The listing builds one solid part. Answer for the finished solid, in the listing's coordinates (mm). A direction names the side the tool comes from. Coordinates: 2 decimals unless noted, no trailing zeros. Order: outer loops, then holes, each group sorted by start corner. A loop starts at its lowest first (then second) coordinate and runs counter-clockwise, first axis right, second up. Notation, with made-up numbers: (77.5, 75.25) - (93.5, 75.25) arc R15 ccw to (93.5, 98.25) - close; hole circle Ø2 at (76.25, -30). An arc over 180 degrees is marked (long way). Use a Markdown table: item, result. Add a question column.
Item 1: Find the intervals of material crossed by line 1 along X through (y, z) = (-6.75, -6.5); line 2 along X through (y, z) = (-0.5, -10); line 3 along Z through (x, y) = (-9, 16.75), in increasing order.
Item 2: Flat-ended cylindrical pins translate along their axes: P1, Ø2, axis at x = -8.5, y = -4.5, coming from the -Z side; P2, Ø5, axis at x = -2, z = -6.5, coming from the +Y side; P3, Ø4, axis at x = 9.5, z = -1, coming from the -Y side; P4, Ø2, axis at y = 11.5, z = 0.5, coming from the -X side. Find the tip coordinate at first contact, or state that the pin passes through.
Item 3: The part is cut by section C-C, the plane x = 11.5. Give the vertices of the cut face in (y, z).
Item 4: The part is cut by section D-D, the plane z = -3. Give the vertices of the cut face in (x, y).
Item 5: The part is cut by section A-A, the plane y = 11. Give the vertices of the cut face in (x, z).
Item 6: For faces 4 (the flat face through (14.99, -0.83, -2.73)), 5 (the flat face through (19.014, -7, -3)), 6 (the flat face through (11.014, -7, -3)), 7 (the flat face through (12, -6.45, -3)), determine the directions among +Z, -Z, +X, -X, +Y, -Y from which every point of the face is accessible in a straight line to the end or side of a thin tool.
Item 7: The mould has two halves that part along X. Classify faces 1 (the flat face through (-10, -7, -8)), 2 (the flat face through (18.014, 9, 0)), 3 (the flat face through (8.989, 18.924, 0.479)): released by +X, released by -X, zero draft, split by the parting line, or undercut.
Item 8: The part is cut by section B-B, the plane z = -0.25. Give the vertices of the cut face in (x, y) (3 decimals).
from build123d import *

# Parameters (mm, degrees)
EXTRUDE_1_DEPTH      = 2
EXTRUDE_1_DEPTH_BACK = 1
BOSS_EXTRUDE1_DEPTH  = 10
LPATTERN1_COUNT      = 2
LPATTERN1_PITCH      = 25
SKETCH2_W            = 3
SKETCH2_H            = 4
BOSS_EXTRUDE2_DEPTH  = 14
BOSS_EXTRUDE3_DEPTH  = 4
LPATTERN2_COUNT      = 2
LPATTERN2_PITCH      = 25
CUT_EXTRUDE1_DEPTH   = 10


with BuildPart() as part:
    # Эскиз2 → Бобышка-Вытянуть1 (new, two sides: drawn at the far end of the back side and taken through both)
    with BuildSketch(Plane.XY.offset(-EXTRUDE_1_DEPTH_BACK)):
        Polygon((18.01429863, 0), (18.01429863, 26.7), (-11.98570137, 26.7), (-11.98570137, -2.25), (18.01429863, -2.25), align=None)
    extrude(amount=EXTRUDE_1_DEPTH + EXTRUDE_1_DEPTH_BACK)

    # Sketch1 → Boss-Extrude1 (add)
    with BuildSketch(Plane.XY.offset(2)):
        with BuildLine():
            Line((-5.98570137, -6.45), (-7.98570137, -6.45))
            Line((-7.98570137, -6.45), (-7.98570137, -2.25))
            Line((-7.98570137, -2.25), (-11.98570137, -2.25))
            Line((-11.98570137, -2.25), (-11.98570137, -6.45))
            Line((-11.98570137, -6.45), (-13.98570137, -6.45))
            Line((-13.98570137, -6.45), (-13.98570137, -7.45))
            ThreePointArc((-13.98570137, -7.45), (-13.399914932, -8.864213562), (-11.98570137, -9.45))
            Line((-11.98570137, -9.45), (-7.98570137, -9.45))
            ThreePointArc((-7.98570137, -9.45), (-6.571487808, -8.864213562), (-5.98570137, -7.45))
            Line((-5.98570137, -7.45), (-5.98570137, -6.45))
        make_face()
    boss_extrude1 = extrude(amount=-BOSS_EXTRUDE1_DEPTH)

    # LPattern1: Boss-Extrude1 ×2
    with Locations(*[(i * LPATTERN1_PITCH, 0, 0) for i in range(1, LPATTERN1_COUNT)]):
        add(boss_extrude1)

    # Sketch2 → Boss-Extrude2 (add)
    with BuildSketch(Plane(origin=(0, 0, 2), x_dir=(-1, 0, 0), z_dir=(0, 0, -1))):
        with Locations((-9.283605158, -0.25)):
            Rectangle(SKETCH2_W, SKETCH2_H)
    extrude(amount=BOSS_EXTRUDE2_DEPTH)

    # Sketch3 → Boss-Extrude3 (add)
    with BuildSketch(Plane.ZY.offset(-13.01429863)):
        Polygon((-4.5, -2.25), (-1, -2.25), (-1, 0.558861968), align=None)
    boss_extrude3 = extrude(amount=-BOSS_EXTRUDE3_DEPTH)

    # LPattern2: Boss-Extrude3 ×2
    with Locations(*[(-i * LPATTERN2_PITCH, 0, 0) for i in range(1, LPATTERN2_COUNT)]):
        add(boss_extrude3)

    # Sketch4 → Cut-Extrude1 (cut)
    with BuildSketch(Plane(origin=(0, 0, -1), x_dir=(-1, 0, 0), z_dir=(0, 0, -1))):
        with BuildLine():
            Line((-10.321327868, 19.682942102), (-7.619737196, 18.144453997))
            ThreePointArc((-7.619737196, 18.144453997), (-9.751909083, 15.519632814), (-10.51429863, 12.225))
            ThreePointArc((-10.51429863, 12.225), (-3.01429863, 4.725), (4.48570137, 12.225))
            ThreePointArc((4.48570137, 12.225), (3.723311823, 15.519632814), (1.591139935, 18.144453997))
            Line((1.591139935, 18.144453997), (4.292730608, 19.682942102))
            Line((4.292730608, 19.682942102), (13.385264368, 19.682942102))
            Line((13.385264368, 19.682942102), (19.56091022, 30.423181844))
            Line((19.56091022, 30.423181844), (-22.587954431, 29.74009492))
            Line((-22.587954431, 29.74009492), (-18.01429863, 19.682942102))
            Line((-18.01429863, 19.682942102), (-10.321327868, 19.682942102))
        make_face()
    extrude(amount=-CUT_EXTRUDE1_DEPTH, mode=Mode.SUBTRACT)


solid = part.part
Solution:
| question | item | result |
|---|---|---|
| 1 | line 1 | x = -13.99 to -5.99, 11.01 to 19.01 |
| 1 | line 2 | x = 7.78 to 10.78 |
| 1 | line 3 | z = -1 to 2 |
| 2 | P1 | stops at z = -8 |
| 2 | P2 | passes through |
| 2 | P3 | stops at y = -8.76 |
| 2 | P4 | stops at x = -11.99 |
| 3 | outline | (-8.76, -8) - (-6.45, -8) - (-6.45, 2) - (-8.76, 2) - close; (-2.25, -1) - (19.68, -1) - (19.68, 2) - (-2.25, 2) - close |
| 4 | outline | (-13.99, -7.45) arc R2 ccw to (-11.99, -9.45) - (-7.99, -9.45) arc R2 ccw to (-5.99, -7.45) - (-5.99, -6.45) - (-7.99, -6.45) - (-7.99, -1.05) - (-11.99, -1.05) - (-11.99, -6.45) - (-13.99, -6.45) - close; (7.78, -2.25) - (10.78, -2.25) - (10.78, 1.75) - (7.78, 1.75) - close; (11.01, -7.45) arc R2 ccw to (13.01, -9.45) - (17.01, -9.45) arc R2 ccw to (19.01, -7.45) - (19.01, -6.45) - (17.01, -6.45) - (17.01, -1.05) - (13.01, -1.05) - (13.01, -6.45) - (11.01, -6.45) - close |
| 5 | outline | (-11.99, -1) - (-4.38, -1) - (-4.38, 2) - (-11.99, 2) - close; (10.41, -1) - (18.01, -1) - (18.01, 2) - (10.41, 2) - close |
| 6 | face 4 | -Z, +X, +Y |
| 6 | face 5 | +Z, -Z, +X, +Y, -Y |
| 6 | face 6 | +Z, -Z, -Y |
| 6 | face 7 | +Z, -Z |
| 7 | face 1 | zero draft |
| 7 | face 2 | released by +X |
| 7 | face 3 | undercut |
| 8 | outline | (-13.986, -7.45) arc R2 ccw to (-11.986, -9.45) - (-7.986, -9.45) arc R2 ccw to (-5.986, -7.45) - (-5.986, -6.45) - (-7.986, -6.45) - (-7.986, -2.25) - (13.014, -2.25) - (13.014, -6.45) - (11.014, -6.45) - (11.014, -7.45) arc R2 ccw to (13.014, -9.45) - (17.014, -9.45) arc R2 ccw to (19.014, -7.45) - (19.014, -6.45) - (17.014, -6.45) - (17.014, -2.25) - (18.014, -2.25) - (18.014, 19.683) - (10.321, 19.683) - (7.62, 18.144) arc R7.5 cw (long way) to (-1.591, 18.144) - (-4.293, 19.683) - (-11.986, 19.683) - (-11.986, -6.45) - (-13.986, -6.45) - close |
